Autodesk Inventor part; units mm, degrees
ref_plane "YZ Plane" through (0, 0, 0) normal (1, 0, 0) x (0, 1, 0)
ref_plane "XZ Plane" through (0, 0, 0) normal (0, 1, 0) x (-1, 0, 0)
ref_plane "XY Plane" through (0, 0, 0) normal (0, 0, 1) x (1, 0, 0)
sketch "Sketch1" plane through (0, 0, 0) normal (0, 0, 1) x (1, 0, 0)
  line L0 (0, 0) -> (25.4, 0)
  line L1 (25.4, 0) -> (25.4, 25.4)
  line L2 (25.4, 25.4) -> (0, 25.4)
  line L3 (0, 25.4) -> (0, 0)
  line L4 (3.175, 22.225) -> (22.225, 22.225)
  line L5 (22.225, 22.225) -> (22.225, 3.175)
  line L6 (22.225, 3.175) -> (3.175, 3.175)
  line L7 (3.175, 3.175) -> (3.175, 22.225)
  dimension "d0" = 25.4
  dimension "d1" = 25.4
  dimension "d2" = 3.175
extrude "Extrusion1" add sketch "Sketch1" along normal blind 209.55
sketch "Sketch2" plane through (25.4, 0, 0) normal (1, 0, 0) x (0, 0, -1)
  line L0 (0, 0) -> (0, 25.4)
  line L1 (-209.55, 0) -> (-209.55, 25.4)
  line L2 (0, 0) -> (-209.55, 0)
  line L3 (-209.55, 12.7) -> (-196.85, 12.7) construction
  line L4 (0, 12.7) -> (-12.7, 12.7) construction
  circle A0 centre (-196.85, 12.7) radius 3.302
  line L5 (0, 25.4) -> (-209.55, 25.4)
  line L6 (-196.85, 12.7) -> (-12.7, 12.7) construction
  circle A1 centre (-184.5733, 12.7) radius 3.302
  circle A2 centre (-172.2967, 12.7) radius 3.302
  circle A3 centre (-160.02, 12.7) radius 3.302
  circle A4 centre (-147.7433, 12.7) radius 3.302
  circle A5 centre (-135.4667, 12.7) radius 3.302
  circle A6 centre (-123.19, 12.7) radius 3.302
  circle A7 centre (-110.9133, 12.7) radius 3.302
  circle A8 centre (-98.6367, 12.7) radius 3.302
  circle A9 centre (-86.36, 12.7) radius 3.302
  circle A10 centre (-74.0833, 12.7) radius 3.302
  circle A11 centre (-61.8067, 12.7) radius 3.302
  circle A12 centre (-49.53, 12.7) radius 3.302
  circle A13 centre (-37.2533, 12.7) radius 3.302
  circle A14 centre (-24.9767, 12.7) radius 3.302
  circle A15 centre (-12.7, 12.7) radius 3.302
  dimension "d5" = 12.7
  dimension "d7" = 6.604
  dimension "d13" = 209.55
  dimension "d16" = 12.2767
extrude "Extrusion2" cut sketch "Sketch2" against normal through all contours A0 | A1 | A2 | A3 | A4 | A5 | A6 | A7 | A8 | A9 | A10 | A11 | A12 | A13 | A14 | A15
sketch "Sketch3" plane through (0, 0, 0) normal (0, -1, 0) x (1, 0, 0)
  line L0 (0, 0) -> (25.4, 0)
  line L1 (0, 209.55) -> (25.4, 209.55)
  line L2 (12.7, 209.55) -> (12.7, 0) construction
  circle A0 centre (12.7, 196.85) radius 3.302
  circle A1 centre (12.7, 184.5733) radius 3.302
  circle A2 centre (12.7, 172.2967) radius 3.302
  circle A3 centre (12.7, 160.02) radius 3.302
  circle A4 centre (12.7, 147.7433) radius 3.302
  circle A5 centre (12.7, 135.4667) radius 3.302
  circle A6 centre (12.7, 123.19) radius 3.302
  circle A7 centre (12.7, 110.9133) radius 3.302
  circle A8 centre (12.7, 98.6367) radius 3.302
  circle A9 centre (12.7, 86.36) radius 3.302
  circle A10 centre (12.7, 74.0833) radius 3.302
  circle A11 centre (12.7, 61.8067) radius 3.302
  circle A12 centre (12.7, 49.53) radius 3.302
  circle A13 centre (12.7, 37.2533) radius 3.302
  circle A14 centre (12.7, 24.9767) radius 3.302
  circle A15 centre (12.7, 12.7) radius 3.302
  dimension "d21" = 12.7
  dimension "d22" = 209.55
  dimension "d23" = 6.604
  dimension "d26" = 12.2767
extrude "Extrusion3" cut sketch "Sketch3" against normal blind 25.4
equation "\"d26\" = -0.133333 * d21 + 0.0666667 * d22"
properties part number "Chassis Part9 (26x28)" material "Aluminum 6061"
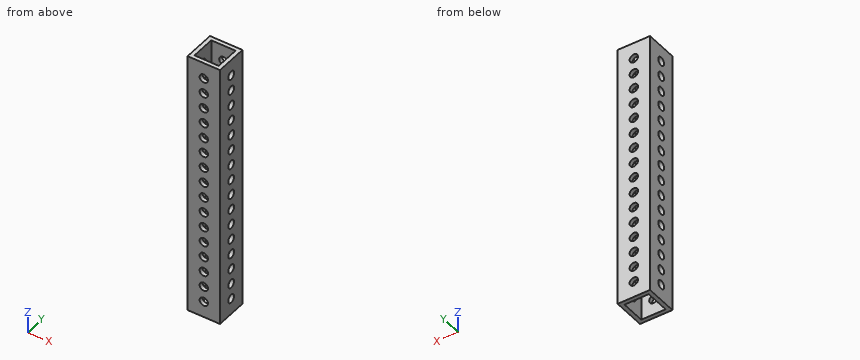
Verification items for the finished model (mm, model axes). Give positions to 0.01 mm unless a question says otherwise; leave off trailing zeros. Write each loop counter-clockwise with the first axis right and the second up, starting at its lowest first coordinate (ties: lowest second). Pieces come first, ordered by that corner, then holes. Notation, with made-up numbers: M 33.25,78 L 63.25,78 A10 cw 63.25,94 Z; hole C 24.5,56 d1. An arc over 180 degrees is marked long. Write item = value, one per line.
(1) Sectioned sample at A-A (x = 19). Record the cut outline in (y, z) (3 decimals), then the cut area to 3 significant figures.
Found:
outline = M 0,0 L 3.175,0 L 3.175,209.55 L 0,209.55 Z; M 22.225,0 L 25.4,0 L 25.4,209.55 L 22.225,209.55 Z
area = 1,330 mm2
(2) Go/stop test with a flat-tipped pin: pin 1 Ø5.5 at (x, z) = (12.7, 160.02) entering from -Y. Record where the tip stops, or that it passes through.
Found:
pin_1 = through
(3) Material ranges on line 1 (Y direction, x = 12.5, z = 92.5) (3 decimals); line 2 (Y direction, x = 0.65, z = 12.7), recorded low to high.
Found:
line_1 = 0 to 3.175, 22.225 to 25.4
line_2 = 0 to 9.4, 16 to 25.4
(4) Sectioned sample at B-B (z = 160.02). Record the cut outline in (x, y) (3 decimals), then the cut area to 3 significant figures.
Found:
outline = M 0,0 L 9.398,0 L 9.398,3.175 L 3.175,3.175 L 3.175,9.398 L 0,9.398 Z; M 0,16.002 L 3.175,16.002 L 3.175,22.225 L 9.398,22.225 L 9.398,25.4 L 0,25.4 Z; M 16.002,0 L 25.4,0 L 25.4,9.398 L 22.225,9.398 L 22.225,3.175 L 16.002,3.175 Z; M 16.002,22.225 L 22.225,22.225 L 22.225,16.002 L 25.4,16.002 L 25.4,25.4 L 16.002,25.4 Z
area = 198 mm2
